Geometry: see drawing. Coordinates: mm, zero at the bounding-box minimum. Round coordinates to 2 decimals unless told otherwise and drop trailing zeros. One line per item, written item: value. Start each with the question number.
1) Section B-B (y = 7.5). State how many separate pieces and enclosed holes the cut face has.
2) Pin query (flat end, axial travel): P1, Ø1.5, axis at x = 18.5, y = 11, coming from the -Z side. Return the tip coordinate at first contact, or that it passes through.
3) Mould query, pull axis X, two halves, no side actions, for the marked faces 1, 2 and 3. Classes: pulls with the +X half, pulls with the -X half, needs draft (parallel to the pull), parting line crosses it, or undercut.
4) Ray query, L1, parallel to Y at x = 18.65, z = 2.3; L2, parallel to X at y = 6.25, z = 2.05; L3, parallel to Y at x = 7.5, z = 2.4. Return the intervals inside material, ascending.
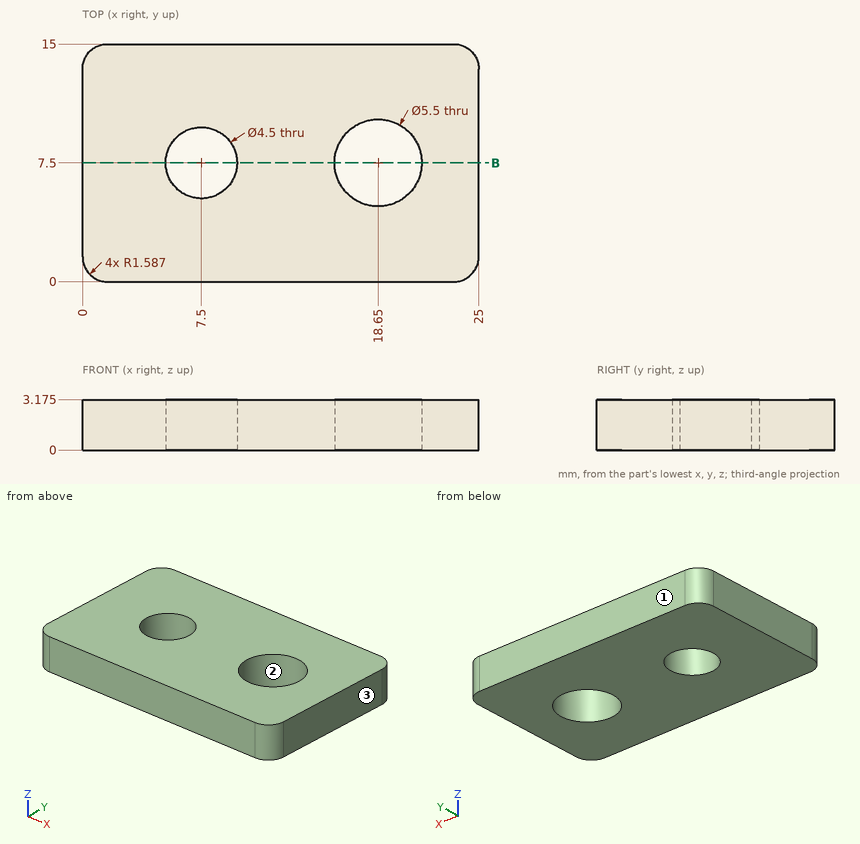
Findings:
1. separate pieces: 3
1. enclosed holes: 0
2. P1: z = 0
3. face 1: needs draft
3. face 2: undercut
3. face 3: pulls with the +X half
4. L1: 0 to 4.75, 10.25 to 15
4. L2: 0 to 5.63, 9.37 to 16.2, 21.1 to 25
4. L3: 0 to 5.25, 9.75 to 15
